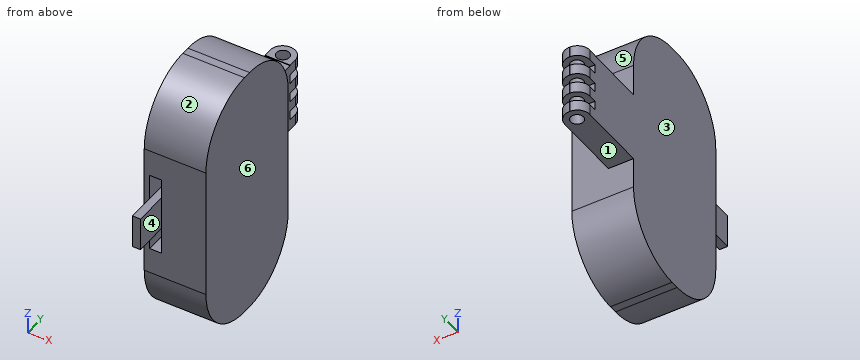
from build123d import *

# Parameters (mm, degrees)
BOSS_EXTRUDE1_DEPTH    = 30
SKETCH4_W              = 12.210528057
SKETCH4_H              = 34
BOSS_EXTRUDE3_DEPTH    = 30
SKETCH5_W              = 12.210528057
SKETCH5_H              = 5.168070784
BOSS_EXTRUDE4_DEPTH    = 10
FILLET1_R              = 6
LPATTERN1_COUNT        = 4
LPATTERN1_PITCH        = 9.7
FILLET1_OF_LPATTERN1_R = 6
SKETCH6_R              = 3.121394117
CUT_EXTRUDE1_DEPTH     = 80.311190797
SKETCH10_W             = 5.758909818
SKETCH10_H             = 38.962624233
CUT_EXTRUDE2_DEPTH     = 35
SKETCH11_W             = 3.89943497
SKETCH11_H             = 16.273957598
BOSS_EXTRUDE5_DEPTH    = 50


with BuildPart() as part:
    # Sketch1 → Boss-Extrude1 (new body)
    with BuildSketch(Plane(origin=(0, 0, 0), x_dir=(0, 0, -1), z_dir=(1, 0, 0))):
        with BuildLine():
            Line((-32.351279839, 31.978308301), (32.351279839, 31.978308301))
            ThreePointArc((32.351279839, 31.978308301), (53.564483275, 23.191511736), (62.351279839, 1.978308301))
            Line((62.351279839, 1.978308301), (62.351279839, -1.978308301))
            ThreePointArc((62.351279839, -1.978308301), (53.564483275, -23.191511736), (32.351279839, -31.978308301))
            Line((32.351279839, -31.978308301), (-32.351279839, -31.978308301))
            ThreePointArc((-32.351279839, -31.978308301), (-53.564483275, -23.191511736), (-62.351279839, -1.978308301))
            Line((-62.351279839, -1.978308301), (-62.351279839, 1.978308301))
            ThreePointArc((-62.351279839, 1.978308301), (-53.564483275, 23.191511736), (-32.351279839, 31.978308301))
        make_face()
    extrude(amount=BOSS_EXTRUDE1_DEPTH)

    # Sketch4 → Boss-Extrude3 (add)
    with BuildSketch(Plane(origin=(0, 31.978308301, 0), x_dir=(1, 0, 0), z_dir=(0, 1, 0))):
        with Locations((6.105264029, 0.308159826)):
            Rectangle(SKETCH4_W, SKETCH4_H)
    extrude(amount=BOSS_EXTRUDE3_DEPTH)

    # Sketch5 → Boss-Extrude4 (add)
    with BuildSketch(Plane(origin=(0, 61.978308301, 0), x_dir=(1, 0, 0), z_dir=(0, 1, 0))):
        with Locations((6.105264029, 14.724124434)):
            Rectangle(SKETCH5_W, SKETCH5_H)
    boss_extrude4 = extrude(amount=BOSS_EXTRUDE4_DEPTH)

    # Fillet1
    fillet1_edges = [part.edges().sort_by_distance(p)[0] for p in [
        (0, 71.978308301, -14.724124434),
        (12.210528057, 71.978308301, -14.724124434),
    ]]
    fillet(fillet1_edges, radius=FILLET1_R)

    # LPattern1: Boss-Extrude4 ×4
    with Locations(*[(0, 0, i * LPATTERN1_PITCH) for i in range(1, LPATTERN1_COUNT)]):
        add(boss_extrude4)

    # Fillet1 of LPattern1
    fillet1_of_lpattern1_edges = [part.edges().sort_by_distance(p)[0] for p in [
        (0, 71.978308301, -5.024124434),
        (12.210528057, 71.978308301, -5.024124434),
        (0, 71.978308301, 4.675875566),
        (12.210528057, 71.978308301, 4.675875566),
        (0, 71.978308301, 14.375875566),
        (12.210528057, 71.978308301, 14.375875566),
    ]]
    fillet(fillet1_of_lpattern1_edges, radius=FILLET1_OF_LPATTERN1_R)

    # Sketch6 → Cut-Extrude1 (cut, through all)
    with BuildSketch(Plane.XY.offset(16.959910958)):
        with Locations((6.210528057, 65.978308301)):
            Circle(SKETCH6_R)
    extrude(amount=-CUT_EXTRUDE1_DEPTH, mode=Mode.SUBTRACT)

    # Sketch10 → Cut-Extrude2 (cut)
    with BuildSketch(Plane.XZ.offset(31.978308301)):
        with Locations((5.551788581, -0.179965931)):
            Rectangle(SKETCH10_W, SKETCH10_H)
    extrude(amount=-CUT_EXTRUDE2_DEPTH, mode=Mode.SUBTRACT)

    # Sketch11 → Boss-Extrude5 (add)
    with BuildSketch(Plane.XZ.offset(-3.021691699)):
        with Locations((5.619023304, 0.398013913)):
            Rectangle(SKETCH11_W, SKETCH11_H)
    extrude(amount=BOSS_EXTRUDE5_DEPTH)


solid = part.part
CAD build for the part. Positions are in the model's coordinates, mm. Face numbers are marked on the shaded views. A direction names the side the tool comes from. Give positions to 0.01 mm unless a question says otherwise; leave off trailing zeros. Write each loop counter-clockwise with the first axis right and the second up, starting at its lowest first coordinate (ties: lowest second). Pieces come first, ordered by that corner, then holes. Notation, with made-up numbers: M -35,30.25 L -10,30.25 A27 ccw -10,54.25 Z; hole C 79,-19 d5. An arc over 180 degrees is marked long. Put each result on its own line as item: value. Start each with the question number.
(1) Mould opens along X. For the marked faces 3, 4, 5 and 6 say: +X half, -X half, draft (parallel to the pull), parting line (faces both ways), or undercut.
(2) Which spindle directions (+Z, -Z, +X, -X, +Y, -Y) get a long thin tool onto all of the face, cutting with end or side? Do the marked faces 1 and 2. Say none if no direction does.
(3) Band-saw the part on B-B, the plane x = 20.75. Write the cut outline in (y, z).
(4) Flat gauge pins, fed straight in: pin 1 Ø3 at (x, y) = (5, -29) entering from -Z; pin 2 Ø7 at (x, y) = (6.21, 65.98) entering from -Z; pin 3 Ø3 at (x, z) = (11.5, -10.5) entering from -Y; pin 4 Ø3.5 at (x, y) = (6.21, 65.98) entering from -Z. Where does each tip first touch, or does it go through?
(5) Probe L1, parallel to X at y = 33.5, z = -2.5; L2, parallel to Z at x = 10.25, y = 56; L3, parallel to Y at x = 18.25, z = -10. List the from-to ranges inside material, lowest first.
(6) Band-saw the part on C-C, the plane z = -22. Write the cut outline in (x, y), and give its area (3 significant figures).
(7) Band-saw the part on D-D, the plane y = 53.5. Write the cut outline in (x, z).
(8) Band-saw the part on A-A, the plane y = -7.5. Write the cut outline in (x, z) (3 decimals).
Response values:
1. face 3: -X half
1. face 4: undercut
1. face 5: draft
1. face 6: +X half
2. face 1: -Z, +X, -X, +Y
2. face 2: +Z, +X, -X, -Y
3. outline: M -31.98,-32.35 A30 ccw -1.98,-62.35 L 1.98,-62.35 A30 ccw 31.98,-32.35 L 31.98,32.35 A30 ccw 1.98,62.35 L -1.98,62.35 A30 ccw -31.98,32.35 Z
4. pin 1: stops at z = -48.12
4. pin 2: stops at z = -17.31
4. pin 3: stops at y = -31.98
4. pin 4: passes through
5. L1: x = 0 to 12.21
5. L2: z = -17.31 to 16.69
5. L3: y = -31.98 to 31.98
6. outline: M 0,-31.98 L 30,-31.98 L 30,31.98 L 0,31.98 Z
6. area: 1,920 mm2
7. outline: M 0,-17.31 L 12.21,-17.31 L 12.21,16.69 L 0,16.69 Z
8. outline: M 0,-61.839 L 30,-61.839 L 30,61.839 L 0,61.839 Z; M 3.669,-7.739 L 7.569,-7.739 L 7.569,8.535 L 3.669,8.535 Z; hole M 2.672,-19.661 L 8.431,-19.661 L 8.431,19.301 L 2.672,19.301 Z
